Can you work these out from the drawing? Everything is in mm from the part's minimum corner. A direction names the side the tool comes from. Give positions to 0.01 mm unless a question says otherwise; leave off trailing zeros. Order: outer loops, then holes, each group sorted by start corner. A loop starts at its lowest first (then second) coordinate and runs counter-clockwise, first axis right, second up. Notation, with made-up numbers: M 66.25,73.25 L 112.25,73.25 A13 ccw 112.25,91.25 Z; hole C -28.5,-21 d7. An arc over 180 degrees is marked long. Answer as a JSON object with one key per item and string values.
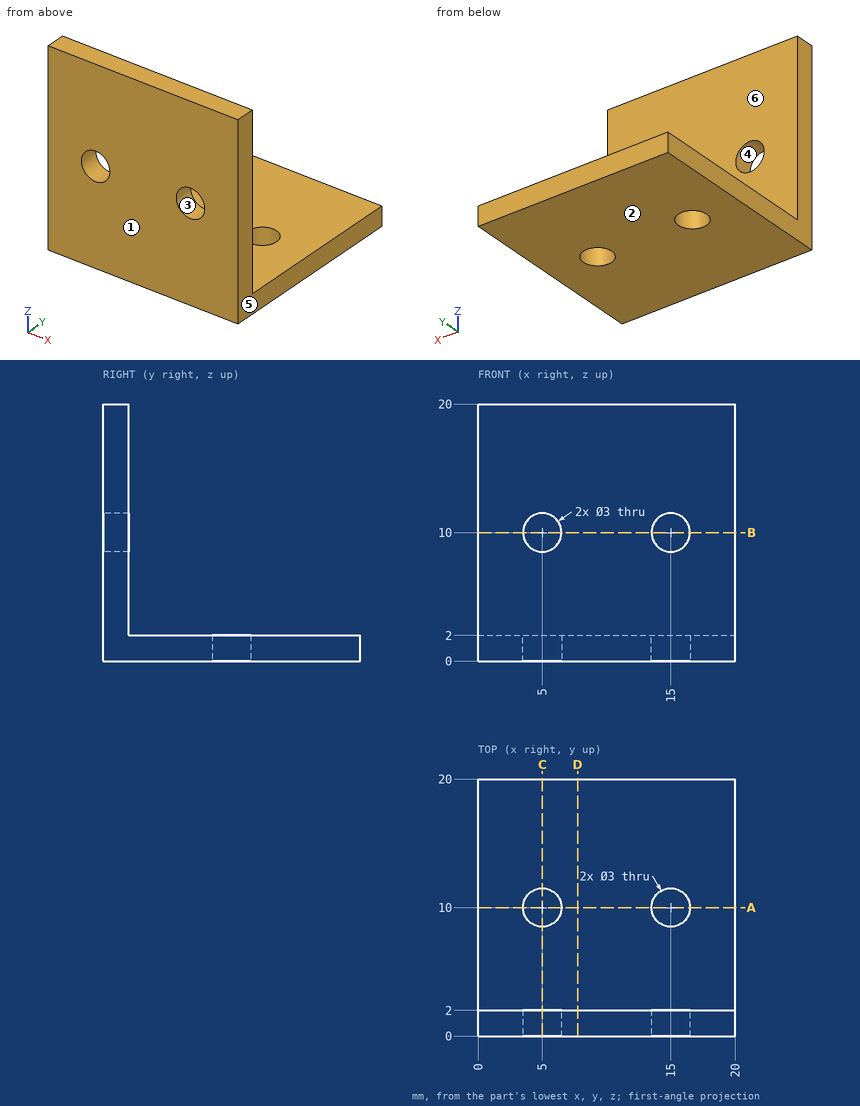
1) For the marked faces 5 and 6, which set-ups out of +Z, -Z, +X, -X, +Y, -Y let a thin tool reach every point of the face, with its end or its side?
Results found:
{"face 5": "+Z, -Z, +X, +Y, -Y", "face 6": "+Z, +X, -X, +Y"}
2) I want a section at D-D on x = 7.75. Write out the boundary of the cut face in (y, z), and give its area (3 significant figures).
Results found:
{"outline": "M 0,0 L 20,0 L 20,2 L 2,2 L 2,20 L 0,20 Z", "area": "76.0 mm²"}
3) I want a section at A-A on y = 10. Write out the boundary of the cut face in (x, z).
Results found:
{"outline": "M 0,0 L 3.5,0 L 3.5,2 L 0,2 Z; M 6.5,0 L 13.5,0 L 13.5,2 L 6.5,2 Z; M 16.5,0 L 20,0 L 20,2 L 16.5,2 Z"}
4) I want a section at C-C on x = 5. Write out the boundary of the cut face in (y, z), and give its area (3 significant figures).
Results found:
{"outline": "M 0,0 L 8.5,0 L 8.5,2 L 2,2 L 2,8.5 L 0,8.5 Z; M 0,11.5 L 2,11.5 L 2,20 L 0,20 Z; M 11.5,0 L 20,0 L 20,2 L 11.5,2 Z", "area": "64.0 mm²"}
5) Thinking about a two-plate mould opening in Z: for the marked faces 1, 2, 3 and 4, which applies, pulls with the +Z half, pulls with the -Z half, needs draft (parallel to the pull), parting line crosses it, or undercut?
Results found:
{"face 1": "needs draft", "face 2": "pulls with the -Z half", "face 3": "undercut", "face 4": "undercut"}
6) I'm going to push flat-ended pins straight in: pin 1 Ø5 at (x, y) = (5, 10) entering from +Z; pin 2 Ø8 at (x, z) = (15.5, 10) entering from -Y; pin 3 Ø9 at (x, z) = (12.5, 14) entering from +Y. Where does each tip first touch, or does it pass through?
Results found:
{"pin 1": "stops at z = 2", "pin 2": "stops at y = 0", "pin 3": "stops at y = 2"}
7) I need wall thicknesses on L1, parallel to Y at x = 15, z = 0.55; L2, parallel to Y at x = 10.75, z = 12. Which ranges of each line are inside material? Lowest first, please.
Results found:
{"L1": "y = 0 to 8.5, 11.5 to 20", "L2": "y = 0 to 2"}
